Could you check a few things on this model? Use its own coordinates, in mm. Coordinates: 2 decimals unless noted, no trailing zeros. Loops run counter-clockwise (first coordinate to the right, second up) from the corner with the lowest first, then second, coordinate; pieces in that order, holes last.
from build123d import *

# Parameters (mm, degrees)
SKETCH1_R           = 0.55
EXTRUDE1_DEPTH      = 66
EXTRUDE1_DEPTH_BACK = 9
SKETCH2_R           = 0.3
EXTRUDE2_DEPTH      = 2
EXTRUDE2_DEPTH_BACK = 0.5


with BuildPart() as part:
    # Sketch1 → Extrude1 (new body, two sides)
    with BuildSketch(Plane(origin=(0, 0, 0), x_dir=(1, 0, 0), z_dir=(0, 1, 0))) as extrude1_sk:
        Circle(SKETCH1_R)
    extrude(amount=EXTRUDE1_DEPTH)
    extrude(extrude1_sk.sketch, amount=-EXTRUDE1_DEPTH_BACK)

    # Sketch2 → Extrude2 (add, two sides)
    with BuildSketch(Plane.XY) as extrude2_sk:
        with Locations((-0.8, 0.3)):
            Circle(SKETCH2_R)
    extrude(amount=EXTRUDE2_DEPTH)
    extrude(extrude2_sk.sketch, amount=-EXTRUDE2_DEPTH_BACK)


solid = part.part
(1) Imagine slicing it at B-B, the plane x = -0.8. Write out the boundary of the cut face in (y, z).
Answers:
outline: (0, -0.5) - (0.6, -0.5) - (0.6, 2) - (0, 2) - close
(2) I need wall thicknesses on probe 1 along Z at (x, y) = (-0.1, 43); probe 2 along Y at (x, z) = (-0.7, 1.15); probe 3 along Y at (x, z) = (-0.55, 0.7). Which ranges of each line are inside material? Lowest first, please.
Answers:
probe 1: z = -0.54 to 0.54
probe 2: y = 0.02 to 0.58
probe 3: y = 0.13 to 0.47
(3) Imagine slicing it at A-A, the plane y = 60. Write out the boundary of the cut face in (x, z), and give its area (3 significant figures).
Answers:
outline: circle Ø1.1 at (0, 0)
area: 0.950 mm2
(4) Imagine slicing it at C-C, the plane z = 1.2. Write out the boundary of the cut face in (x, y).
Answers:
outline: circle Ø0.6 at (-0.8, 0.3)
